Check sheet for the modelled part. Datum: model origin and axes. Units: mm. A direction names the side the tool comes from. Round coordinates to 2 decimals unless told otherwise and drop trailing zeros. Order: outer loops, then holes, each group sorted by start corner. A loop starts at its lowest first (then second) coordinate and runs counter-clockwise, first axis right, second up. Notation, with made-up numbers: (86.25, 43) -> (95.25, 43) arc R17 ccw to (95.25, 61) -> close; hole circle Ø9 at (-2.75, -26.75). An arc over 180 degrees is marked (long way). Answer in a Markdown table with one row per item. Add a question column.
1. Sectioned sample at C-C, the plane z = 30. Record the boundary of the cut face in (x, y) (3 decimals).
2. Depth check by flat-ended pin: P1, Ø5, axis at x = 21.5, y = 6.5, coming from the +Z side; P2, Ø3, axis at x = -5.5, y = 62.5, coming from the -Z side; P3, Ø3.5, axis at y = 34.5, z = -24.5, coming from the +X side; P4, Ø8, axis at y = 53.5, z = -12.5, coming from the -X side. Enter the tip coordinate at first touch or a pass-through.
3. Sectioned sample at A-A, the plane y = 40. Record the boundary of the cut face in (x, z), then the cut area to 3 significant figures.
4. Material ranges on L1, parallel to Y at x = 5, z = 20.25 (3 decimals); L2, parallel to X at y = 0, z = 30 (3 decimals); L3, parallel to Z at x = -12, y = 21, recorded low to high. Write a range as from..to.
5. Access from +Z, -Z, +X, -X, +Y, -Y to the whole of each face (thin tool, end or side, straight path). Record for faces 1 (the flat face through (-11, 36, -26.5)), 2 (the flat face through (7.414, 60.78, 24.429)), 3 (the flat face through (-30, 0, 1)), 4 (the flat face through (6.4, 14.5, -22.3)).
6. Sectioned sample at B-B, the plane x = 20. Record the boundary of the cut face in (y, z) (3 decimals), then the cut area to 3 significant figures.
7. Sectioned sample at D-D, the plane x = 14. Record the boundary of the cut face in (y, z), then the cut area to 3 significant figures.
8. Draft check along Z on faces 5 (the cylindrical face through (-5.374, 11.516, -20.88)), 6 (the flat face through (0, 2.5, -1)), 7 (the flat face through (6.4, 14.5, 22.3)), 8 (the cylindrical face through (18.47, 0.04, 30.8)). Enter one of: +Z half, -Z half, draft (parallel to the pull), parting line (faces both ways), or undercut.
```python
from build123d import *

# Parameters (mm, degrees)
SKETCH1_W           = 60
SKETCH1_H           = 80
BOSS_EXTRUDE1_DEPTH = 2.5
SKETCH2_R           = 1.725
CUT_EXTRUDE1_DEPTH  = 51.249378106
SKETCH3_W           = 50
SKETCH3_H           = 66
BOSS_EXTRUDE2_DEPTH = 7
SKETCH4_W           = 19.9
SKETCH4_H           = 40.6
CUT_EXTRUDE2_DEPTH  = 101.072473738
SKETCH5_R           = 1.725
CUT_EXTRUDE3_DEPTH  = 101.072473738
CUT_EXTRUDE4_DEPTH  = 4.2


with BuildPart() as part:
    # Sketch1 → Boss-Extrude1 (new, symmetric)
    with BuildSketch(Plane(origin=(0, 0, 0), x_dir=(1, 0, 0), z_dir=(0, 1, 0))):
        Rectangle(SKETCH1_W, SKETCH1_H)
    extrude(amount=BOSS_EXTRUDE1_DEPTH, both=True)

    # Sketch2 → Cut-Extrude1 (cut, through all)
    with BuildSketch(Plane(origin=(0, 2.5, 0), x_dir=(1, 0, 0), z_dir=(0, 1, 0))):
        with Locations(Location((-20, 30, 0), (0, 0, 270))):
            Circle(SKETCH2_R)
        with Locations(Location((20, 30, 0), (0, 0, 270))):
            Circle(SKETCH2_R)
        with Locations(Location((20, -30, 0), (0, 0, 270))):
            Circle(SKETCH2_R)
        with Locations(Location((-20, -30, 0), (0, 0, 270))):
            Circle(SKETCH2_R)
    extrude(amount=-CUT_EXTRUDE1_DEPTH, mode=Mode.SUBTRACT)

    # Sketch3 → Boss-Extrude2 (add)
    with BuildSketch(Plane.XY.offset(19.5)):
        with Locations((0, 35.5)):
            Rectangle(SKETCH3_W, SKETCH3_H)
    boss_extrude2 = extrude(amount=BOSS_EXTRUDE2_DEPTH)

    # Mirror1: Boss-Extrude2 across plane
    add(boss_extrude2.mirror(Plane.XY))

    # Sketch4 → Cut-Extrude2 (cut, through all)
    with BuildSketch(Plane.XY.offset(26.5)):
        with Locations((0, 37.7)):
            Rectangle(SKETCH4_W, SKETCH4_H)
    extrude(amount=-CUT_EXTRUDE2_DEPTH, mode=Mode.SUBTRACT)

    # Sketch5 → Cut-Extrude3 (cut, through all)
    with BuildSketch(Plane.XY.offset(26.5)):
        with Locations((-5, 62.2)):
            Circle(SKETCH5_R)
        with Locations((5, 62.2)):
            Circle(SKETCH5_R)
        with Locations((-5, 13.2)):
            Circle(SKETCH5_R)
        with Locations((5, 13.2)):
            Circle(SKETCH5_R)
    extrude(amount=-CUT_EXTRUDE3_DEPTH, mode=Mode.SUBTRACT)

    # Sketch6 → Cut-Extrude4 (cut)
    with BuildSketch(Plane.XY.offset(26.5)):
        Polygon((-1.766838493, 62.2), (-3.383419246, 65), (-6.616580754, 65), (-8.233161507, 62.2), (-6.616580754, 59.4), (-3.383419246, 59.4), align=None)
        Polygon((1.766838493, 62.2), (3.383419246, 59.4), (6.616580754, 59.4), (8.233161507, 62.2), (6.616580754, 65), (3.383419246, 65), align=None)
        Polygon((-1.766838493, 13.2), (-3.383419246, 16), (-6.616580754, 16), (-8.233161507, 13.2), (-6.616580754, 10.4), (-3.383419246, 10.4), align=None)
        Polygon((8.233161507, 13.2), (6.616580754, 16), (3.383419246, 16), (1.766838493, 13.2), (3.383419246, 10.4), (6.616580754, 10.4), align=None)
    cut_extrude4 = extrude(amount=-CUT_EXTRUDE4_DEPTH, mode=Mode.SUBTRACT)

    # Mirror3: Cut-Extrude4 across plane
    add(cut_extrude4.mirror(Plane.XY), mode=Mode.SUBTRACT)


solid = part.part
```
Answer key:
| question | item | result |
|---|---|---|
| 1 | outline | (-30, -2.5) -> (-21.725, -2.5) -> (-21.725, 2.5) -> (-30, 2.5) -> close; (-18.275, -2.5) -> (18.275, -2.5) -> (18.275, 2.5) -> (-18.275, 2.5) -> close; (21.725, -2.5) -> (30, -2.5) -> (30, 2.5) -> (21.725, 2.5) -> close |
| 2 | P1 | stops at z = 26.5 |
| 2 | P2 | stops at z = -22.3 |
| 2 | P3 | stops at x = 25 |
| 2 | P4 | passes through |
| 3 | outline | (-25, -26.5) -> (-9.95, -26.5) -> (-9.95, -19.5) -> (-25, -19.5) -> close; (-25, 19.5) -> (-9.95, 19.5) -> (-9.95, 26.5) -> (-25, 26.5) -> close; (9.95, -26.5) -> (25, -26.5) -> (25, -19.5) -> (9.95, -19.5) -> close; (9.95, 19.5) -> (25, 19.5) -> (25, 26.5) -> (9.95, 26.5) -> close |
| 3 | area | 421 mm² |
| 4 | L1 | y = -2.5..11.475, 14.925..17.4, 58..60.475, 63.925..68.5 |
| 4 | L2 | x = -30..-21.725, -18.275..18.275, 21.725..30 |
| 4 | L3 | z = -26.5..-19.5, 19.5..26.5 |
| 5 | face 1 | -Z, +X, -X, +Y |
| 5 | face 2 | +Z |
| 5 | face 3 | +Z, -Z, -X, +Y, -Y |
| 5 | face 4 | -Z |
| 6 | outline | (-2.5, -40) -> (2.5, -40) -> (2.5, -31.725) -> (-2.5, -31.725) -> close; (-2.5, -28.275) -> (2.5, -28.275) -> (2.5, -26.5) -> (68.5, -26.5) -> (68.5, -19.5) -> (2.5, -19.5) -> (2.5, 19.5) -> (68.5, 19.5) -> (68.5, 26.5) -> (2.5, 26.5) -> (2.5, 28.275) -> (-2.5, 28.275) -> close; (-2.5, 31.725) -> (2.5, 31.725) -> (2.5, 40) -> (-2.5, 40) -> close |
| 6 | area | 1,290 mm² |
| 7 | outline | (-2.5, -40) -> (2.5, -40) -> (2.5, -26.5) -> (68.5, -26.5) -> (68.5, -19.5) -> (2.5, -19.5) -> (2.5, 19.5) -> (68.5, 19.5) -> (68.5, 26.5) -> (2.5, 26.5) -> (2.5, 40) -> (-2.5, 40) -> close |
| 7 | area | 1,320 mm² |
| 8 | face 5 | draft |
| 8 | face 6 | undercut |
| 8 | face 7 | +Z half |
| 8 | face 8 | undercut |
